The listing builds one solid part. Answer for the finished solid, in the listing's coordinates (mm). A direction names the side the tool comes from. Round coordinates to 2 decimals unless told otherwise and drop trailing zeros. Loops run counter-clockwise (first coordinate to the right, second up) from the corner with the lowest first, then second, coordinate; pieces in that order, holes last. Notation, with made-up numbers: (-26.5, 55) -> (31.5, 55) arc R23 cw to (31.5, 84) -> close; hole circle Ø3 at (-7.75, 13.5). An arc over 180 degrees is marked (long way). Use a Markdown table: item, result. Add a question column.
Q1. Which of the six approach directions +Z, -Z, +X, -X, +Y, -Y give full straight-line access (tool end or side, diameter ignored) to faces 1 (the flat face through (16, -14, -80)), 2 (the flat face through (420, 22, -209)), 3 (the flat face through (212.644, -14.93, -247.217))?
Q2. Consider line 1 (X direction, y = 49, z = -129); line 2 (Z direction, x = 107, y = 14); line 3 (Y direction, x = 260.5, z = -11.5). Determine where each line is inside the solid, lowest interval first.
Q3. For a pull along X with two mould halves and no side action, classify faces 4 (the flat face through (405, -10, -85)), 5 (the flat face through (105, 19, -280)), 6 (the cylindrical face through (412.395, 25.89, -53.844)) as released by +X, released by -X, zero draft, split by the parting line, or undercut.
Q4. Section C-C on x = 255.5 is taken. Give the vertices of the cut face in (y, z).
Q5. Given pin 1 Ø16 at (y, z) = (-2.5, -174.5) entering from +X; pin 2 Ø16 at (x, y) = (65, -5.5) entering from -Z; pin 3 Ø12 at (y, z) = (38.5, -11) entering from +X; pin 4 Ø11 at (x, y) = (246, -17) entering from +Z, each flat-ended and moving along its own axis, determine where each tip first touches the part or whether it passes through.
Q6. Section A-A on x = 14.5 is taken. Give the vertices of the cut face in (y, z), then the cut area to 3 significant figures.
Q7. Section B-B on z = -164.5 is taken. Give the number of separate pieces and of enclosed holes in the cut face, then the cut area to 3 significant figures.
from build123d import *

# Parameters (mm, degrees)
SKETCH_2_W          = 416.5
SKETCH_2_H          = 300
EXTRUDE_1_DEPTH     = 60
EXTRUDE_4_DEPTH     = 5
SKETCH_5_R          = 12
EXTRUDE_3_DEPTH     = 20
SKETCH_8_W          = 260
SKETCH_8_H          = 10
EXTRUDE_5_DEPTH     = 15
EXTRUDE_6_DEPTH     = 5
EXTRUDE_START       = 5
EXTRUDE_8_DEPTH     = 5
EXTRUDE_START_2     = 20
SKETCH_10_R         = 12
EXTRUDE_7_DEPTH     = 20
SKETCH_13_W         = 260
SKETCH_13_H         = 10
EXTRUDE_10_DEPTH    = 15
SKETCH_14_W         = 260
SKETCH_14_H         = 10
EXTRUDE_11_DEPTH    = 5
SKETCH_15_W         = 386.5
SKETCH_15_H         = 300
CUT_EXTRUDE_2_DEPTH = 40
SKETCH_16_R         = 26.25
CUT_EXTRUDE_3_DEPTH = 10
SKETCH_17_W         = 386.5
SKETCH_17_H         = 300
CUT_EXTRUDE_4_DEPTH = 10
EXTRUDE_12_DEPTH    = 30
SKETCH_19_W         = 386.5
SKETCH_19_H         = 346.960050319
CUT_EXTRUDE_5_DEPTH = 20
SKETCH_20_R         = 3
EXTRUDE_13_DEPTH    = 5
SKETCH_22_R         = 3
EXTRUDE_14_DEPTH    = 5
EXTRUDE_15_DEPTH    = 5
SKETCH_24_W         = 52.5
SKETCH_24_H         = 76.5
CUT_EXTRUDE_6_DEPTH = 10
EXTRUDE_16_DEPTH    = 52.5
FILLET_1_R          = 5


with BuildPart() as part:
    # 草图2 → 凸台-拉伸1 (new body)
    with BuildSketch(Plane(origin=(0, 0, 0), x_dir=(1, 0, 0), z_dir=(0, 1, 0))):
        with Locations((191.75, 130)):
            Rectangle(SKETCH_2_W, SKETCH_2_H)
    extrude(amount=EXTRUDE_1_DEPTH)

    # 草图6 → 凸台-拉伸4 (add)
    with BuildSketch(Plane(origin=(400, 0, 0), x_dir=(0, 0, -1), z_dir=(1, 0, 0))):
        with BuildLine():
            Line((15, 10), (0, 10))
            Line((0, 10), (0, 0))
            Line((0, 0), (260, 0))
            Line((260, 0), (260, 10))
            Line((260, 10), (245, 10))
            Line((245, 10), (232.041510818, 41.100582022))
            ThreePointArc((232.041510818, 41.100582022), (215, 52.461618456), (197.958489182, 41.100582022))
            Line((197.958489182, 41.100582022), (185, 10))
            Line((185, 10), (170, 10))
            Line((170, 10), (90, 10))
            Line((90, 10), (75, 10))
            Line((75, 10), (62.041510818, 41.100582022))
            ThreePointArc((62.041510818, 41.100582022), (45, 52.461618456), (27.958489182, 41.100582022))
            Line((27.958489182, 41.100582022), (15, 10))
        make_face()
    extrude(amount=EXTRUDE_4_DEPTH)

    # 草图5 → 凸台-拉伸3 (add)
    with BuildSketch(Plane(origin=(400, 0, 0), x_dir=(0, 0, -1), z_dir=(1, 0, 0))):
        with Locations((215, 34)):
            Circle(SKETCH_5_R)
        with Locations(Location((45, 34, 0), (0, 0, 180))):
            Circle(SKETCH_5_R)
    extrude(amount=EXTRUDE_3_DEPTH)

    # 草图8 → 凸台-拉伸5 (add)
    with BuildSketch(Plane(origin=(405, 0, 0), x_dir=(0, 0, -1), z_dir=(1, 0, 0))):
        with Locations((130, 5)):
            Rectangle(SKETCH_8_W, SKETCH_8_H)
    extrude(amount=EXTRUDE_5_DEPTH)

    # 草图9 → 凸台-拉伸6 (add)
    with BuildSketch(Plane(origin=(420, 0, 0), x_dir=(0, 0, -1), z_dir=(1, 0, 0))):
        with BuildLine():
            Line((15, 10), (27.958489182, 41.100582022))
            ThreePointArc((27.958489182, 41.100582022), (45, 52.461618456), (62.041510818, 41.100582022))
            Line((62.041510818, 41.100582022), (75, 10))
            Line((75, 10), (185, 10))
            Line((185, 10), (197.958489182, 41.100582022))
            ThreePointArc((197.958489182, 41.100582022), (215, 52.461618456), (232.041510818, 41.100582022))
            Line((232.041510818, 41.100582022), (245, 10))
            Line((245, 10), (260, 10))
            Line((260, 10), (260, 0))
            Line((260, 0), (0, 0))
            Line((0, 0), (0, 10))
            Line((0, 10), (15, 10))
        make_face()
    extrude(amount=EXTRUDE_6_DEPTH)

    # 草图11 → 凸台-拉伸8 (add)
    with BuildSketch(Plane.ZY.offset(16.5).offset(EXTRUDE_START)):
        with BuildLine():
            Line((-245, 10), (-260, 10))
            Line((-260, 10), (-260, 0))
            Line((-260, 0), (0, 0))
            Line((0, 0), (0, 10))
            Line((0, 10), (-15, 10))
            Line((-15, 10), (-27.958489182, 41.100582022))
            ThreePointArc((-27.958489182, 41.100582022), (-45, 52.461618456), (-62.041510818, 41.100582022))
            Line((-62.041510818, 41.100582022), (-75, 10))
            Line((-75, 10), (-90, 10))
            Line((-90, 10), (-170, 10))
            Line((-170, 10), (-185, 10))
            Line((-185, 10), (-197.958489182, 41.100582022))
            ThreePointArc((-197.958489182, 41.100582022), (-215, 52.461618456), (-232.041510818, 41.100582022))
            Line((-232.041510818, 41.100582022), (-245, 10))
        make_face()
    extrude(amount=-EXTRUDE_8_DEPTH)

    # 草图10 → 凸台-拉伸7 (add)
    with BuildSketch(Plane.ZY.offset(16.5).offset(EXTRUDE_START_2)):
        with Locations((-45, 34)):
            Circle(SKETCH_10_R)
        with Locations(Location((-215, 34, 0), (0, 0, 180))):
            Circle(SKETCH_10_R)
    extrude(amount=-EXTRUDE_7_DEPTH)

    # 草图13 → 凸台-拉伸10 (add)
    with BuildSketch(Plane.ZY.offset(21.5)):
        with Locations((-130, 5)):
            Rectangle(SKETCH_13_W, SKETCH_13_H)
    extrude(amount=EXTRUDE_10_DEPTH)

    # 草图14 → 凸台-拉伸11 (add)
    with BuildSketch(Plane.ZY.offset(36.5).offset(EXTRUDE_START)):
        with Locations((-130, 5)):
            Rectangle(SKETCH_14_W, SKETCH_14_H)
        with BuildLine():
            Line((-232.041510818, 41.100582022), (-245, 10))
            Line((-245, 10), (-185, 10))
            Line((-185, 10), (-197.958489182, 41.100582022))
            ThreePointArc((-197.958489182, 41.100582022), (-215, 52.461618456), (-232.041510818, 41.100582022))
        make_face()
        with BuildLine():
            Line((-75, 10), (-15, 10))
            Line((-15, 10), (-27.958489182, 41.100582022))
            ThreePointArc((-27.958489182, 41.100582022), (-45, 52.461618456), (-62.041510818, 41.100582022))
            Line((-62.041510818, 41.100582022), (-75, 10))
        make_face()
    extrude(amount=-EXTRUDE_11_DEPTH)

    # 草图15 → 切除-拉伸2 (cut)
    with BuildSketch(Plane(origin=(0, 60, 0), x_dir=(1, 0, 0), z_dir=(0, 1, 0))):
        with Locations((191.75, 130)):
            Rectangle(SKETCH_15_W, SKETCH_15_H)
    extrude(amount=-CUT_EXTRUDE_2_DEPTH, mode=Mode.SUBTRACT)

    # 草图16 → 切除-拉伸3 (cut)
    with BuildSketch(Plane(origin=(0, 20, 0), x_dir=(1, 0, 0), z_dir=(0, 1, 0))):
        with Locations(Location((303.75, 35, 0), (0, 0, 270))):
            Circle(SKETCH_16_R)
        with Locations(Location((247.75, 35, 0), (0, 0, 270))):
            Circle(SKETCH_16_R)
        with Locations(Location((191.75, 35, 0), (0, 0, 270))):
            Circle(SKETCH_16_R)
        with Locations(Location((135.75, 35, 0), (0, 0, 270))):
            Circle(SKETCH_16_R)
        with Locations(Location((79.75, 35, 0), (0, 0, 270))):
            Circle(SKETCH_16_R)
        with Locations(Location((219.75, 83.497422612, 0), (0, 0, 270))):
            Circle(SKETCH_16_R)
        with Locations(Location((275.75, 83.497422612, 0), (0, 0, 270))):
            Circle(SKETCH_16_R)
        with Locations(Location((163.75, 83.497422612, 0), (0, 0, 270))):
            Circle(SKETCH_16_R)
        with Locations(Location((107.75, 83.497422612, 0), (0, 0, 270))):
            Circle(SKETCH_16_R)
        with Locations(Location((191.75, 131.994845224, 0), (0, 0, 270))):
            Circle(SKETCH_16_R)
        with Locations(Location((247.75, 131.994845224, 0), (0, 0, 270))):
            Circle(SKETCH_16_R)
        with Locations(Location((135.75, 131.994845224, 0), (0, 0, 270))):
            Circle(SKETCH_16_R)
        with Locations(Location((163.75, 180.492267836, 0), (0, 0, 270))):
            Circle(SKETCH_16_R)
        with Locations(Location((219.75, 180.492267836, 0), (0, 0, 270))):
            Circle(SKETCH_16_R)
        with Locations(Location((191.75, 228.989690448, 0), (0, 0, 270))):
            Circle(SKETCH_16_R)
    extrude(amount=-CUT_EXTRUDE_3_DEPTH, mode=Mode.SUBTRACT)

    # 草图17 → 切除-拉伸4 (cut)
    with BuildSketch(Plane.XZ):
        with Locations((191.75, -130)):
            Rectangle(SKETCH_17_W, SKETCH_17_H)
    extrude(amount=-CUT_EXTRUDE_4_DEPTH, mode=Mode.SUBTRACT)

    # 草图18 → 凸台-拉伸12 (add)
    with BuildSketch(Plane.XZ.offset(-10)):
        Polygon((385, -200), (239.904930741, -200), (303.413460352, -90), (385, -90), (405, -90), (405, -80), (385, -80), (309.186963044, -80), (346.546460718, -15.291451884), (350.876587737, -7.791451884), (41.283666301, -7.791451884), (32.623412263, -7.791451884), (74.313036956, -80), (-1.5, -80), (-21.5, -80), (-21.5, -90), (-1.5, -90), (80.086539648, -90), (143.595069259, -200), (-1.5, -200), (-21.5, -200), (-21.5, -210), (-1.5, -210), (149.368571951, -210), (187.419872981, -275.906786679), (191.75, -283.406786679), (234.131428049, -210), (385, -210), (405, -210), (405, -200), align=None)
        Polygon((86.75, -12.791451884), (342.216333699, -12.791451884), (309.460384119, -69.526420807), (191.75, -273.406786679), (74.039615881, -69.526420807), (41.283666301, -12.791451884), align=None, mode=Mode.SUBTRACT)
    extrude(amount=EXTRUDE_12_DEPTH)

    # 草图19 → 切除-拉伸5 (cut)
    with BuildSketch(Plane.XZ.offset(-10)):
        with Locations((191.75, -153.48002516)):
            Rectangle(SKETCH_19_W, SKETCH_19_H)
    extrude(amount=CUT_EXTRUDE_5_DEPTH, mode=Mode.SUBTRACT)

    # 草图20 → 凸台-拉伸13 (add)
    with BuildSketch(Plane(origin=(-1.5, 0, 0), x_dir=(0, 0, -1), z_dir=(1, 0, 0))):
        with Locations(Location((95, 30, 0), (0, 0, 180))):
            Circle(SKETCH_20_R)
        with Locations(Location((210, 30, 0), (0, 0, 180))):
            Circle(SKETCH_20_R)
    extrude(amount=EXTRUDE_13_DEPTH)

    # 草图22 → 凸台-拉伸14 (add)
    with BuildSketch(Plane.ZY.offset(-385).offset(EXTRUDE_START)):
        with Locations((-95, 30)):
            Circle(SKETCH_22_R)
        with Locations((-210, 30)):
            Circle(SKETCH_22_R)
    extrude(amount=-EXTRUDE_14_DEPTH)

    # 草图23 → 凸台-拉伸15 (add)
    with BuildSketch(Plane(origin=(3.5, 0, 0), x_dir=(0, 0, -1), z_dir=(1, 0, 0))):
        Polygon((95, 30), (96.13137085, 28.86862915), (99.313351365, 32.050609665), (97.050609665, 34.313351365), (93.86862915, 31.13137085), align=None)
    extrude(amount=-EXTRUDE_15_DEPTH)

    # 草图24 → 切除-拉伸6 (cut)
    with BuildSketch(Plane(origin=(0, 20, 0), x_dir=(1, 0, 0), z_dir=(0, 1, 0))):
        with Locations((295.75, 241.75)):
            Rectangle(SKETCH_24_W, SKETCH_24_H)
    extrude(amount=-CUT_EXTRUDE_6_DEPTH, mode=Mode.SUBTRACT)

    # 草图25 → 凸台-拉伸16 (add)
    with BuildSketch(Plane.ZY.offset(-322)):
        Polygon((-203.5, 20), (-272.782032303, -20), (-255.461524227, -20), (-203.5, 10), align=None)
    extrude(amount=EXTRUDE_16_DEPTH)

    # 圆角1
    fillet_1_edges = [part.edges().sort_by_distance(p)[0] for p in [
        (295.75, 20, -203.5),
    ]]
    fillet(fillet_1_edges, radius=FILLET_1_R)


solid = part.part
Checked values:
| question | item | result |
|---|---|---|
| 1 | face 1 | -X, -Y |
| 1 | face 2 | none |
| 1 | face 3 | -Z, -Y |
| 2 | line 1 | x = -16.5 to -1.5, 385 to 400 |
| 2 | line 2 | z = -280 to -109.74, -57.26 to 20 |
| 2 | line 3 | y = -20 to -10, 10 to 20 |
| 3 | face 4 | released by +X |
| 3 | face 5 | zero draft |
| 3 | face 6 | undercut |
| 4 | outline | (-20, -210) -> (-10, -210) -> (-10, -200) -> (-20, -200) -> close; (-20, -172.99) -> (-10, -172.99) -> (-10, -162.99) -> (-20, -162.99) -> close; (-20, -12.79) -> (-10, -12.79) -> (-10, -7.79) -> (-20, -7.79) -> close; (10, -280) -> (20, -280) -> (20, -157.07) -> (10, -157.07) -> close; (10, -106.91) -> (20, -106.91) -> (20, -100.2) -> (10, -100.2) -> close; (10, -66.79) -> (20, -66.79) -> (20, -60.08) -> (10, -60.08) -> close; (10, -9.92) -> (20, -9.92) -> (20, 20) -> (10, 20) -> close |
| 5 | pin 1 | stops at x = 425 |
| 5 | pin 2 | stops at z = -210 |
| 5 | pin 3 | stops at x = 400 |
| 5 | pin 4 | stops at z = -7.79 |
| 6 | outline | (-20, -210) -> (-10, -210) -> (-10, -200) -> (-20, -200) -> close; (-20, -90) -> (-10, -90) -> (-10, -80) -> (-20, -80) -> close; (10, -280) -> (20, -280) -> (20, 20) -> (10, 20) -> close |
| 6 | area | 3,200 mm2 |
| 7 | separate pieces | 5 |
| 7 | enclosed holes | 0 |
| 7 | area | 5,450 mm2 |
